Input: part model. Units: mm. Frame: model coordinates. Face numbers are marked on the shaded views. A direction names the side the tool comes from. Coordinates: 2 decimals unless noted, no trailing zeros. Loops run counter-clockwise (first coordinate to the right, second up) from the corner with the lowest first, then second, coordinate; pieces in that order, holes last. Notation, with made-up numbers: (60, 29.25) - (112, 29.25) arc R34 ccw to (112, 60.25) - close; hole circle Ø3 at (-2.5, -11). An arc over 180 degrees is marked (long way). Use one line per item in the form item = value.
Autodesk Inventor part; units mm, degrees
ref_plane "YZ Plane" through (0, 0, 0) normal (1, 0, 0) x (0, 1, 0)
ref_plane "XZ Plane" through (0, 0, 0) normal (0, 1, 0) x (-1, 0, 0)
ref_plane "XY Plane" through (0, 0, 0) normal (0, 0, 1) x (1, 0, 0)
sketch "Sketch1" plane through (0, 0, 0) normal (0, 0, 1) x (1, 0, 0)
  line L0 (-5.2, 1.7) -> (5.2, 1.7)
  line L1 (5.2, 1.7) -> (5.2, -1.7)
  line L2 (5.2, -1.7) -> (-5.2, -1.7)
  line L3 (-5.2, -1.7) -> (-5.2, 1.7)
  line L4 (-5.2, 1.7) -> (5.2, -1.7) construction
  line L5 (5.2, 1.7) -> (-5.2, -1.7) construction
  line L6 (0, 0) -> (0, -7.5)
  circle A0 centre (0, -7.5) radius 2.6
  line L7 (-6, 2.5) -> (6, 2.5)
  line L8 (6, 2.5) -> (6, -2.5)
  line L9 (6, -2.5) -> (-6, -2.5)
  line L10 (-6, -2.5) -> (-6, 2.5)
  line L11 (-6, 2.5) -> (6, -2.5) construction
  line L12 (6, 2.5) -> (-6, -2.5) construction
  circle A1 centre (0, -7.5) radius 2.8
  line L13 (-6, -2.5) -> (-2.4445, -8.8654)
  line L14 (6, -2.5) -> (2.4445, -8.8654)
  line L15 (0, -7.5) -> (2.1964, -10.1176)
  line L16 (0, -7.5) -> (3.417, -7.5) construction
  line L17 (0, -7.5) -> (-2.5132, -10.4951)
  line L18 (0, -7.5) -> (3.9099, -7.5) construction
  line L19 (2.4445, -8.8654) -> (1.9255, -9.7947)
  line L20 (-2.4445, -8.8654) -> (-1.9255, -9.7947)
  line L21 (-1.9255, -9.7947) -> (-2.4397, -8.3988)
  line L22 (1.9255, -9.7947) -> (2.4397, -8.3988)
  point P0 (-2.2345, -8.8294)
  point P1 (2.2345, -8.8294)
  point P2 (-2.5783, -7.8348)
  point P3 (2.5783, -7.8348)
  dimension "d0" = 10.4
  dimension "d1" = 3.4
  dimension "d2" = 7.5
  dimension "d3" = 5.2
  dimension "d4" = 12
  dimension "d5" = 5
  dimension "d9" = 5.6
  dimension "d10" = 50
  dimension "d11" = 130
extrude "Extrusion1" add sketch "Sketch1" along normal blind 6 contours L9 L10 L7 L8 | L9 L14 A1 L6 | L6 A1 L13 L9 | A1 L22 A0 L6 | L6 A0 L21 A1 | A1 L21 L20 | L19 L22 A1
fillet "Fillet1" radius 2 4 edges at (-6, 2.5, 3) (6, 2.5, 3) (-6, -2.5, 3) (6, -2.5, 3)
fillet "Fillet2" radius 0.1 2 edges at (-1.9255, -9.7947, 3) (1.9255, -9.7947, 3)
fillet "Fillet3" radius 0.8 4 edges at (5.2, -1.7, 3) (5.2, 1.7, 3) (-5.2, -1.7, 3) (-5.2, 1.7, 3)
properties part number "Turret_Holder_2_test_pt2"
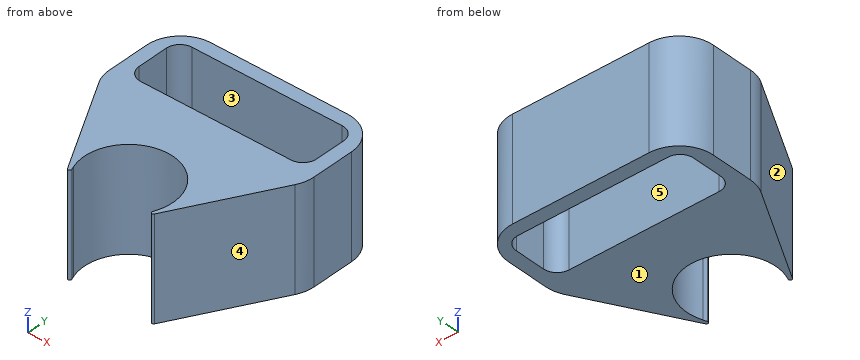
Q1. Ray query, line 1 along Y through (x, z) = (0, 3); line 2 along X through (y, z) = (0, 1); line 3 along X through (y, z) = (-7.5, 4.35). Return the intervals inside material, ascending. Write a range as [from, to].
Check values:
line_1 = [-4.9, -1.7], [1.7, 2.5]
line_2 = [-6, -5.2], [5.2, 6]
line_3 = [-3.21, -2.6], [2.6, 3.21]
Q2. Pull-direction query (X, two-part tool) for the marked faces 1, 2 and 3; classes: pulls with the +X half, pulls with the -X half, needs draft (parallel to the pull), parting line crosses it, or undercut.
Check values:
face_1 = needs draft
face_2 = pulls with the -X half
face_3 = undercut
Q3. Cut plane C-C, the plane y = -3.5. Return loops of the section in (x, z).
Check values:
outline = (-5.44, 0) - (5.44, 0) - (5.44, 6) - (-5.44, 6) - close
Q4. First-contact query: P1, Ø6, axis at x = 0, y = -7.5, coming from the +Z side; P2, Ø2, axis at y = -5, z = 0.5, coming from the +X side; P3, Ø1.5, axis at y = -4, z = 4, coming from the +X side. Flat tips, straight axial feed; report the tip coordinate or a pass-through.
Check values:
P1 = 6
P2 = 5.16
P3 = 5.58
Q5. Cut plane A-A, the plane x = 0. Return loops of the section in (y, z), then the cut area to 3 significant figures.
Check values:
outline = (-4.9, 0) - (-1.7, 0) - (-1.7, 6) - (-4.9, 6) - close; (1.7, 0) - (2.5, 0) - (2.5, 6) - (1.7, 6) - close
area = 24.0 mm²
Q6. Set-up query: the marked faces 4 and 5. Return all of +Z, -Z, +X, -X, +Y, -Y with unobstructed straight access to the full face (end or side cutting, diameter ignored); none if empty.
Check values:
face_4 = +Z, -Z, +X, -Y
face_5 = +Z, -Z
Q7. Cut plane B-B, the plane y = -7.5. Return loops of the section in (x, z), then the cut area to 3 significant figures.
Check values:
outline = (-3.21, 0) - (-2.6, 0) - (-2.6, 6) - (-3.21, 6) - close; (2.6, 0) - (3.21, 0) - (3.21, 6) - (2.6, 6) - close
area = 7.29 mm²
